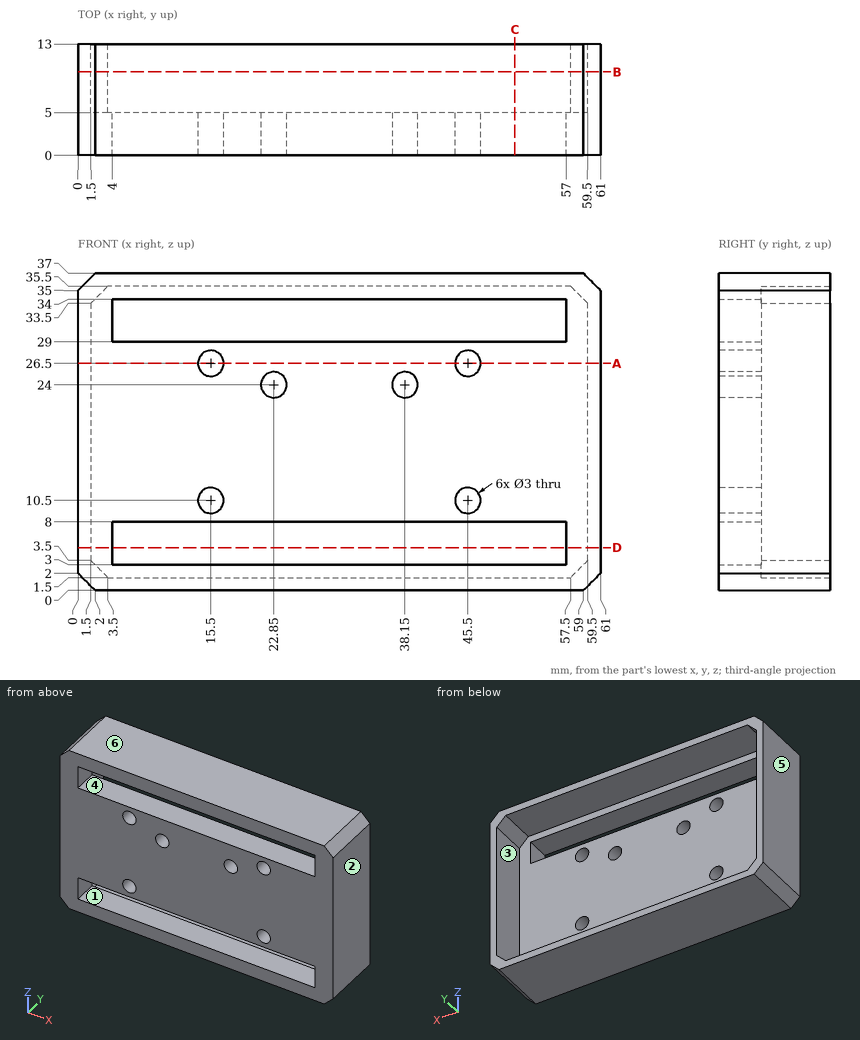
Design review of the part shown in the three views and the two pictorial views. Dimensions are in mm from the part's minimum x, y and z. A direction names the side the tool comes from. Coordinates: 2 decimals unless noted, no trailing zeros. Order: outer loops, then holes, each group sorted by start corner. A loop starts at its lowest first (then second) coordinate and runs counter-clockwise, first axis right, second up.
Item 1: The part is to be moulded in two halves that separate along X. For the marked faces 4, 5 and 6, say which applies: pulls with the +X half, pulls with the -X half, needs draft (parallel to the pull), parting line crosses it, or undercut.
Item 2: Take a section at C-C, the plane x = 51. Write out the cut boundary in (y, z).
Item 3: For the marked faces 1, 2 and 3, list the 3-axis set-ups (+Z, -Z, +X, -X, +Y, -Y) from which the entire face can be reached by the end or side of a thin tool; tool diameter is ignored.
Item 4: For pin 1 Ø5 at (x, z) = (45.5, 26.5) entering from +Y; pin 2 Ø2.5 at (x, z) = (38.15, 24) entering from -Y, all flat-tipped, find the tip position at first contact; note any pin that passes through.
Item 5: For line 1 (Z direction, x = 45.5, y = 3.15); line 2 (X direction, y = 11, z = 3); line 3 (Z direction, x = 46.5, y = 6), list the stretches that pass through material, from the lowest coordinate up.
Item 6: Take a section at D-D, the plane z = 5. Write out the cut boundary in (x, y).
Item 7: Take a section at B-B, the plane y = 9.75. Write out the cut boundary in (x, z), then the cut area to 3 significant figures.
Item 8: Take a section at A-A, the plane z = 26.5. Write out the cut boundary in (x, y).
The answers:
1. face 4: undercut
1. face 5: pulls with the -X half
1. face 6: needs draft
2. outline: (0, 0) - (13, 0) - (13, 1.5) - (5, 1.5) - (5, 3) - (0, 3) - close; (0, 8) - (5, 8) - (5, 29) - (0, 29) - close; (0, 34) - (5, 34) - (5, 35.5) - (13, 35.5) - (13, 37) - (0, 37) - close
3. face 1: +Y, -Y
3. face 2: +Z, -Z, +X, +Y, -Y
3. face 3: +Y
4. pin 1: stops at y = 5
4. pin 2: passes through
5. line 1: z = 0 to 3, 8 to 9, 12 to 25, 28 to 29, 34 to 37
5. line 2: x = 0 to 2, 59 to 61
5. line 3: z = 0 to 1.5, 35.5 to 37
6. outline: (0, 0) - (4, 0) - (4, 5) - (1.5, 5) - (1.5, 13) - (0, 13) - close; (57, 0) - (61, 0) - (61, 13) - (59.5, 13) - (59.5, 5) - (57, 5) - close
7. outline: (0, 2) - (2, 0) - (59, 0) - (61, 2) - (61, 35) - (59, 37) - (2, 37) - (0, 35) - close; hole (1.5, 3.5) - (3.5, 1.5) - (57.5, 1.5) - (59.5, 3.5) - (59.5, 33.5) - (57.5, 35.5) - (3.5, 35.5) - (1.5, 33.5) - close
7. area: 285 mm2
8. outline: (0, 0) - (14, 0) - (14, 5) - (1.5, 5) - (1.5, 13) - (0, 13) - close; (17, 0) - (44, 0) - (44, 5) - (17, 5) - close; (47, 0) - (61, 0) - (61, 13) - (59.5, 13) - (59.5, 5) - (47, 5) - close
